Can you work these out from the drawing? Everything is in mm from the part's minimum corner. A direction names the side the tool comes from. Round coordinates to 2 decimals unless told otherwise and drop trailing zeros. Write each loop counter-clockwise with the first axis right and the second up, starting at its lowest first coordinate (ties: lowest second). Pieces come first, ordered by that corner, then holes. Notation, with made-up numbers: M 67,-23.5 L 119,-23.5 A20 cw 119,5.5 Z; hole C 70.5,40.25 d7. An arc over 180 degrees is marked long. Answer in a Markdown table with one row per item. Add a question column.
(1) Suppose I cut it at D-D, the plane y = 14.75. Write out the boundary of the cut face in (x, z), then the cut area to 3 significant figures.
(2) I'm going to push flat-ended pins straight in: pin 1 (6 mm diameter, centred on y = 2, z = 5, fed in from +X); pin 2 (8 mm diameter, centred on x = 10.5, y = 6, fed in from +Z); pin 3 (1.5 mm diameter, centred on y = 13, z = 7.5, fed in from -X). Where does each tip first touch, or does it pass through?
(3) Suppose I cut it at A-A, the plane z = 9. Write out the boundary of the cut face in (x, y), then the cut area to 3 significant figures.
(4) Suppose I cut it at C-C, the plane y = 1.5. Write out the boundary of the cut face in (x, z), then the cut area to 3 significant figures.
(5) If we mould it in two halves opening along X, with no side actions, what happens to the marked faces 3, 4 and 5? For each: released by +X, released by -X, zero draft, split by the parting line, or undercut.
(6) Suppose I cut it at B-B, the plane x = 9. Write out the boundary of the cut face in (y, z), then the cut area to 3 significant figures.
(7) For the marked faces 1 and 2, which set-ups out of +Z, -Z, +X, -X, +Y, -Y let a thin tool reach every point of the face, with its end or its side?
(8) If I drill on probe 1 along Z at (x, y) = (9, 7.5); probe 2 along Z at (x, y) = (10, 2); probe 3 along X at (y, z) = (14.5, 9.5), over which ranges is the centre line in solid material (lowest first)?
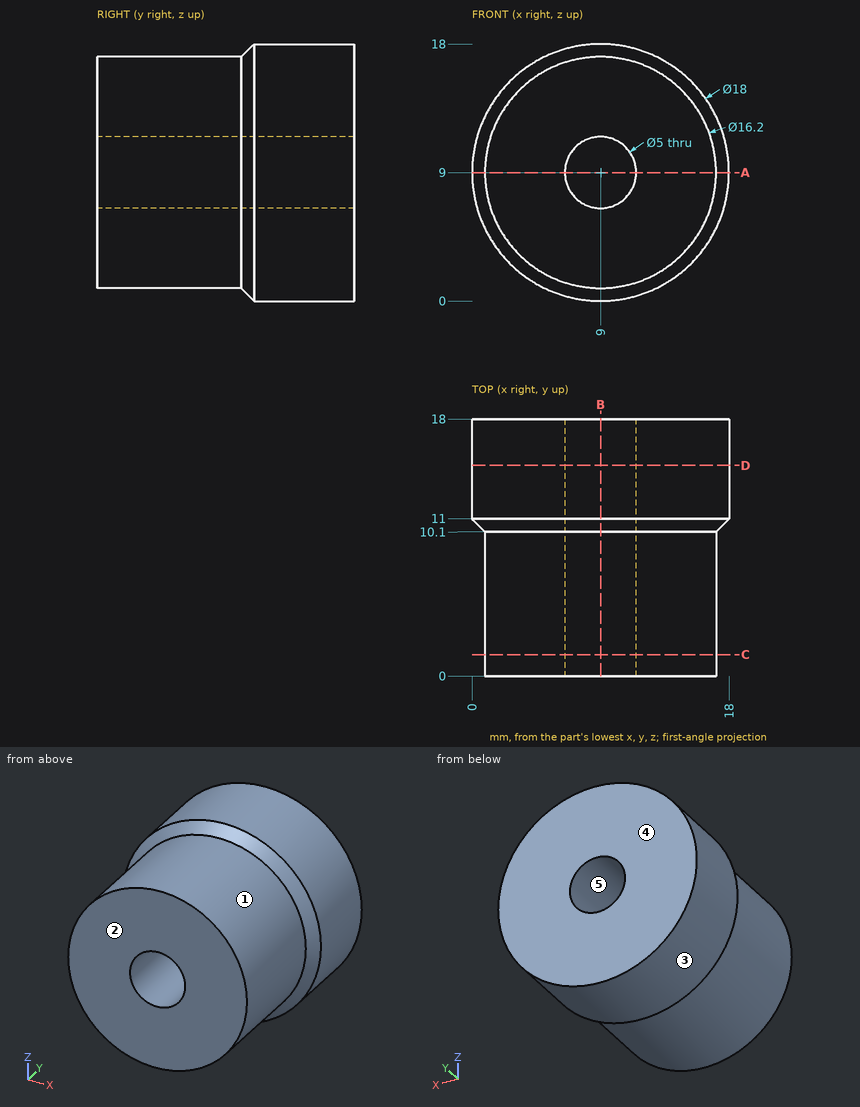
Calculated:
| question | item | result |
|---|---|---|
| 1 | outline | C 9,9 d18; hole C 9,9 d5 |
| 1 | area | 235 mm² |
| 2 | pin 1 | x = 17.04 |
| 2 | pin 2 | z = 17.1 |
| 2 | pin 3 | x = 0.03 |
| 3 | outline | M 0,11 L 0.9,10.1 L 0.9,0 L 6.5,0 L 6.5,18 L 0,18 Z; M 11.5,0 L 17.1,0 L 17.1,10.1 L 18,11 L 18,18 L 11.5,18 Z |
| 3 | area | 215 mm² |
| 4 | outline | C 9,9 d16.2; hole C 9,9 d5 |
| 4 | area | 186 mm² |
| 5 | face 3 | split by the parting line |
| 5 | face 4 | zero draft |
| 5 | face 5 | undercut |
| 6 | outline | M 0,0.9 L 10.1,0.9 L 11,0 L 18,0 L 18,6.5 L 0,6.5 Z; M 0,11.5 L 18,11.5 L 18,18 L 11,18 L 10.1,17.1 L 0,17.1 Z |
| 6 | area | 215 mm² |
| 7 | face 1 | -Y |
| 7 | face 2 | +Z, -Z, +X, -X, -Y |
| 8 | probe 1 | 0.9 to 6.5, 11.5 to 17.1 |
| 8 | probe 2 | 0.96 to 6.71, 11.29 to 17.04 |
| 8 | probe 3 | 0.01 to 6.55, 11.45 to 17.99 |
